from build123d import *

# Parameters (mm, degrees)
F1_DEPTH = 2
F2_R     = 1


with BuildPart() as f1:
    # F0 (on Front) → F1 (new body)
    with BuildSketch(Plane.XZ):
        with BuildLine():
            ThreePointArc((21.4, 3.9), (20.989949, 4.889949), (20, 5.3))
            ThreePointArc((20, 5.3), (19.010051, 2.910051), (21.4, 3.9))
        make_face()
        Polygon((0, 3.9), (0, 0), (40, 0), (40, 3.9), (40, 7.8), (20, 7.8), (0, 7.8), align=None)
        with BuildLine():
            ThreePointArc((6.4, 3.9), (5, 2.5), (3.6, 3.9))
            ThreePointArc((3.6, 3.9), (5, 5.3), (6.4, 3.9))
        make_face(mode=Mode.SUBTRACT)
        with BuildLine():
            ThreePointArc((21.4, 3.9), (19.010051, 2.910051), (20, 5.3))
            ThreePointArc((20, 5.3), (20.989949, 4.889949), (21.4, 3.9))
        make_face(mode=Mode.SUBTRACT)
        with BuildLine():
            ThreePointArc((33.6, 3.9), (35, 5.3), (36.4, 3.9))
            ThreePointArc((36.4, 3.9), (35, 2.5), (33.6, 3.9))
        make_face(mode=Mode.SUBTRACT)
    extrude(amount=F1_DEPTH)

    # F2
    f2_edges = [f1.edges().sort_by_distance(p)[0] for p in [
        (0, -1, 7.8),
        (0, -1, 0),
        (40, -1, 7.8),
        (40, -1, 0),
    ]]
    fillet(f2_edges, radius=F2_R)


solid = f1.part
Source: CAD feature listing. Evaluate the final solid. Frame: model axes, mm. Coordinates: 2 decimals unless noted, no trailing zeros. Loops run counter-clockwise (first coordinate to the right, second up) from the corner with the lowest first, then second, coordinate; pieces in that order, holes last. Notation, with made-up numbers: (-6, -3.5) - (2, -3.5) arc R15 ccw to (2, 18.5) - close; hole circle Ø8 at (87.25, 2.25). An arc over 180 degrees is marked (long way). Return JSON: item names as keys, results as strings.
Q1. Section B-B, the plane y = -1.3. Return loops of the section in (x, z), plus the area to 3 significant figures.
Results:
{"outline": "(0, 1) arc R1 ccw to (1, 0) - (39, 0) arc R1 ccw to (40, 1) - (40, 6.8) arc R1 ccw to (39, 7.8) - (1, 7.8) arc R1 ccw to (0, 6.8) - close; hole circle Ø2.8 at (5, 3.9); hole (20, 5.3) arc R1.4 ccw (long way) to (21.4, 3.9) arc R1.4 ccw to start; hole circle Ø2.8 at (35, 3.9)", "area": "293 mm2"}
Q2. Section A-A, the plane x = 35. Return loops of the section in (y, z).
Results:
{"outline": "(-2, 0) - (0, 0) - (0, 2.5) - (-2, 2.5) - close; (-2, 5.3) - (0, 5.3) - (0, 7.8) - (-2, 7.8) - close"}
Q3. Material intervals for line 1 along Z through (x, y) = (35, -0.4); line 2 along X through (y, z) = (-1.25, 3); line 3 along X through (y, z) = (-0.1, 5), sorted ascending.
Results:
{"line 1": "0 to 2.5, 5.3 to 7.8", "line 2": "0 to 3.93, 6.07 to 18.93, 21.07 to 33.93, 36.07 to 40", "line 3": "0 to 4.13, 5.87 to 19.13, 20.87 to 34.13, 35.87 to 40"}
Q4. Mould query, pull axis X, two halves, no side actions, for faces 1 (the cylindrical face through (33.6, -0.99, 3.84)), 2 (the cylindrical face through (4.35, -0.99, 2.66)), 3 (the cylindrical face through (0.301, -1.014, 0.285)), 4 (the flat face through (20, -2, 6)). Classes: released by +X, released by -X, zero draft, split by the parting line, or undercut.
Results:
{"face 1": "undercut", "face 2": "undercut", "face 3": "released by -X", "face 4": "zero draft"}
Q5. Section D-D, the plane x = 4. Return loops of the section in (y, z).
Results:
{"outline": "(-2, 0) - (0, 0) - (0, 2.92) - (-2, 2.92) - close; (-2, 4.88) - (0, 4.88) - (0, 7.8) - (-2, 7.8) - close"}
Q6. Contact query for a flat-ended pin moving along its axis: P1, Ø2.5, axis at x = 20, z = 3.9, coming from the +Y side (3 decimals). Output: stop coordinate, or through.
Results:
{"P1": "through"}
Q7. Section C-C, the plane z = 3.25. Return loops of the section in (x, y), plus the area to 3 significant figures.
Results:
{"outline": "(0, -2) - (3.76, -2) - (3.76, 0) - (0, 0) - close; (6.24, -2) - (18.76, -2) - (18.76, 0) - (6.24, 0) - close; (21.24, -2) - (33.76, -2) - (33.76, 0) - (21.24, 0) - close; (36.24, -2) - (40, -2) - (40, 0) - (36.24, 0) - close", "area": "65.1 mm2"}
